from build123d import *

# Parameters (mm, degrees)
SKETCH1_R           = 1
BOSS_EXTRUDE1_DEPTH = 22
SKETCH2_R           = 1.5
BOSS_EXTRUDE2_DEPTH = 1


with BuildPart() as part:
    # Sketch1 → Boss-Extrude1 (new body)
    with BuildSketch(Plane(origin=(0, 0, 0), x_dir=(1, 0, 0), z_dir=(0, 1, 0))):
        with Locations(Location((0, 0, 0), (0, 0, 270))):
            Circle(SKETCH1_R)
    extrude(amount=BOSS_EXTRUDE1_DEPTH)

    # Sketch2 → Boss-Extrude2 (add)
    with BuildSketch(Plane.XZ):
        with Locations(Location((0, 0, 0), (0, 0, 270))):
            Circle(SKETCH2_R)
    boss_extrude2 = extrude(amount=BOSS_EXTRUDE2_DEPTH)

    # Mirror2: Boss-Extrude2 across plane
    add(boss_extrude2.mirror(Plane.ZX.offset(11)))


solid = part.part
Design review of the part built by this model. Coordinates are the model's own, in mm. Coordinates: 2 decimals unless noted, no trailing zeros. Order: outer loops, then holes, each group sorted by start corner. A loop starts at its lowest first (then second) coordinate and runs counter-clockwise, first axis right, second up. Notation, with made-up numbers: M 12.5,35 L 33.5,35 A9 cw 33.5,41 Z; hole C 5.5,31 d3. An arc over 180 degrees is marked long. Use a Markdown table: item, result.
(1) Add section B-B (z = 0). Give the boundary of the cut face in (x, y).
Worked answers:
| item | result |
|---|---|
| outline | M -1.5,-1 L 1.5,-1 L 1.5,0 L 1,0 L 1,22 L 1.5,22 L 1.5,23 L -1.5,23 L -1.5,22 L -1,22 L -1,0 L -1.5,0 Z |
(2) Add section A-A (x = 0). Give the boundary of the cut face in (y, z), then the cut area to 3 significant figures.
Worked answers:
| item | result |
|---|---|
| outline | M -1,-1.5 L 0,-1.5 L 0,-1 L 22,-1 L 22,-1.5 L 23,-1.5 L 23,1.5 L 22,1.5 L 22,1 L 0,1 L 0,1.5 L -1,1.5 Z |
| area | 50.0 mm2 |
(3) Wall thickness on probe 1 along Y at (x, z) = (-0.05, -1.4); probe 2 along Z at (x, y) = (0.05, 15.75); probe 3 along X at (y, z) = (20.5, 0.1): over which ranges is each line inside the solid? List them lowest first.
Worked answers:
| item | result |
|---|---|
| probe 1 | y = -1 to 0, 22 to 23 |
| probe 2 | z = -1 to 1 |
| probe 3 | x = -0.99 to 0.99 |
(4) Add section C-C (y = 5.75). Give the boundary of the cut face in (x, z).
Worked answers:
| item | result |
|---|---|
| outline | C 0,0 d2 |
(5) Draft analysis for pull direction Y (two halves, no side actions). For faces 1 (the cylindrical face through (-1, 11, 0)), 2 (the flat face through (0, 23, 0)), 3 (the cylindrical face through (0.45, 22.49, -1.43)), 4 (the flat face through (0, -1, 0)), state which applies: released by +Y, released by -Y, zero draft, split by the parting line, or undercut.
Worked answers:
| item | result |
|---|---|
| face 1 | undercut |
| face 2 | released by +Y |
| face 3 | zero draft |
| face 4 | released by -Y |
